Verification items for this drawing (mm, ordinates from the low corner). Round coordinates to 2 decimals unless told otherwise and drop trailing zeros. Loops run counter-clockwise (first coordinate to the right, second up) from the corner with the lowest first, then second, coordinate; pieces in that order, holes last. Notation, with made-up numbers: (78, 52.25) -> (116, 52.25) arc R16 ccw to (116, 62.25) -> close; hole circle Ø8 at (-39.5, 80.5). An arc over 180 degrees is marked (long way). One line per item, written item: value. Start each with the question number.
1. Material ranges on L1, parallel to X at y = 1.25, z = 62; L2, parallel to X at y = 9.5, z = 79.5; L3, parallel to Z at x = 32.5, y = 8.25, recorded low to high.
2. Release check for a two-part mould opening along X. For the marked faces 1 and 2 record: +X half, -X half, draft (parallel to the pull), parting line (faces both ways), or undercut.
3. Cross-section at B-B on z = 78. Record the cut outline in (x, y).
4. Cross-section at C-C on y = 7. Record the cut outline in (x, z).
5. Cross-section at D-D on z = 27. Record the cut outline in (x, y).
6. Go/stop test with flat-tipped pins: pin 1 (25 mm diameter, centred on x = 47, z = 22.5, fed in from -Y); pin 2 (4 mm diameter, centred on y = 1.5, z = 21.5, fed in from -X); pin 3 (1.5 mm diameter, centred on y = 2.5, z = 31.5, fed in from +X). Record where each tip stops, or that it passes through.
7. Cross-section at A-A on x = 51.5. Record the cut outline in (y, z), then the cut area to 4 significant figures.
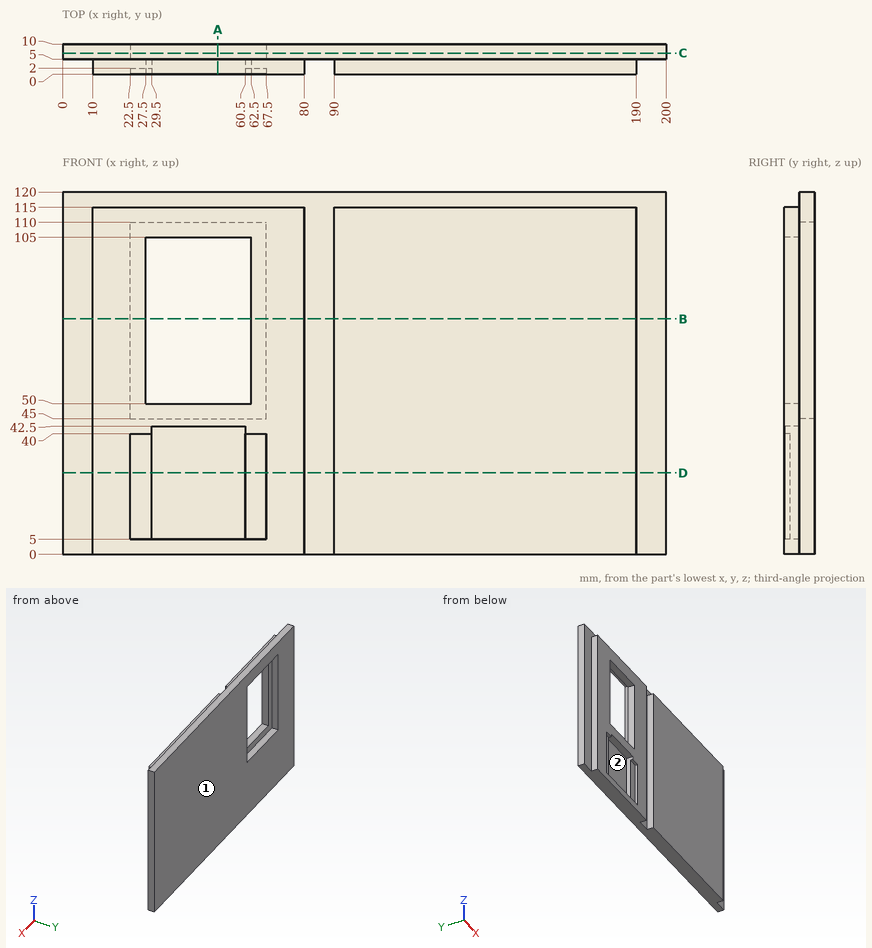
Taken from the geometry:
1. L1: x = 10 to 27.5, 62.5 to 80, 90 to 190
1. L2: x = 0 to 22.5, 67.5 to 200
1. L3: z = 0 to 45, 110 to 120
2. face 1: draft
2. face 2: undercut
3. outline: (0, 5) -> (10, 5) -> (10, 0) -> (27.5, 0) -> (27.5, 5) -> (22.5, 5) -> (22.5, 10) -> (0, 10) -> close; (62.5, 0) -> (80, 0) -> (80, 5) -> (90, 5) -> (90, 0) -> (190, 0) -> (190, 5) -> (200, 5) -> (200, 10) -> (67.5, 10) -> (67.5, 5) -> (62.5, 5) -> close
4. outline: (0, 0) -> (200, 0) -> (200, 120) -> (0, 120) -> close; hole (22.5, 45) -> (67.5, 45) -> (67.5, 110) -> (22.5, 110) -> close
5. outline: (0, 5) -> (10, 5) -> (10, 0) -> (22.5, 0) -> (22.5, 2) -> (29.5, 2) -> (29.5, 5) -> (60.5, 5) -> (60.5, 2) -> (67.5, 2) -> (67.5, 0) -> (80, 0) -> (80, 5) -> (90, 5) -> (90, 0) -> (190, 0) -> (190, 5) -> (200, 5) -> (200, 10) -> (0, 10) -> close
6. pin 1: stops at y = 5
6. pin 2: stops at x = 10
6. pin 3: stops at x = 190
7. outline: (0, 0) -> (10, 0) -> (10, 45) -> (5, 45) -> (5, 50) -> (0, 50) -> (0, 42.5) -> (5, 42.5) -> (5, 5) -> (0, 5) -> close; (0, 105) -> (5, 105) -> (5, 110) -> (10, 110) -> (10, 120) -> (5, 120) -> (5, 115) -> (0, 115) -> close
7. area: 387.5 mm2
